```python
from build123d import *

# Parameters (mm, degrees)
BOSS_EXTRUDE1_DEPTH         = 119.0625
F_1_4_20_TAPPED_HOLE2_D     = 5.1054
F_1_4_20_TAPPED_HOLE2_DEPTH = 16.51
F_1_4_20_TAPPED_HOLE2_TIP   = 1.533816902
F_10_32_TAPPED_HOLE1_D      = 4.0386
F_10_32_TAPPED_HOLE1_DEPTH  = 13.6144
F_10_32_TAPPED_HOLE1_TIP    = 1.213317848


with BuildPart() as part:
    # Sketch1 → Boss-Extrude1 (new body)
    with BuildSketch(Plane.XY):
        Polygon((0, 7.332348419), (-6.35, 3.666174209), (-6.35, -3.666174209), (0, -7.332348419), (6.35, -3.666174209), (6.35, 3.666174209), align=None)
    extrude(amount=BOSS_EXTRUDE1_DEPTH)

    # 1/4-20 Tapped Hole2
    with Locations(Plane(origin=(0, 0, 0), x_dir=(-1, 0, 0), z_dir=(0, 0, -1))):
        with Locations((0, 0)):
            Hole(F_1_4_20_TAPPED_HOLE2_D / 2, depth=F_1_4_20_TAPPED_HOLE2_DEPTH)
            with Locations((0, 0, -(F_1_4_20_TAPPED_HOLE2_DEPTH + F_1_4_20_TAPPED_HOLE2_TIP / 2))):  # 118° drill point
                Cone(0, F_1_4_20_TAPPED_HOLE2_D / 2, F_1_4_20_TAPPED_HOLE2_TIP, mode=Mode.SUBTRACT)

    # #10-32 Tapped Hole1
    with Locations(Plane.XY.offset(119.0625)):
        with Locations((0, 0)):
            Hole(F_10_32_TAPPED_HOLE1_D / 2, depth=F_10_32_TAPPED_HOLE1_DEPTH)
            with Locations((0, 0, -(F_10_32_TAPPED_HOLE1_DEPTH + F_10_32_TAPPED_HOLE1_TIP / 2))):  # 118° drill point
                Cone(0, F_10_32_TAPPED_HOLE1_D / 2, F_10_32_TAPPED_HOLE1_TIP, mode=Mode.SUBTRACT)


solid = part.part
```
Geometry check sheet. Reference: the model listing, model coordinates, mm. A direction names the side the tool comes from. Coordinates: 2 decimals unless noted, no trailing zeros. Order: outer loops, then holes, each group sorted by start corner. A loop starts at its lowest first (then second) coordinate and runs counter-clockwise, first axis right, second up.
Item 1: Scan lines: line 1 along X through (y, z) = (0, 116); line 2 along Y through (x, z) = (0, 115); line 3 along X through (y, z) = (0, 11). Record each from-to range of solid material in increasing order.
Item 2: Section check A-A (z = 92.5). Enter the section's corners in (x, y), plus the area to 3 significant figures.
Item 3: Mould release check, pull along X, two halves, no side actions. Record for faces 4 (the conical face through (-0.42, 0.13, 17.78)), 5 (the flat face through (-3.131, 5.525, 58.698)), 6 (the flat face through (3.219, 5.474, 58.698)): released by +X, released by -X, zero draft, split by the parting line, or undercut.
Item 4: Tool access check on faces 1 (the flat face through (1, -2, 119.062)), 2 (the cylindrical face through (2.435, 0.767, 8.371)), 3 (the cylindrical face through (-1.926, 0.607, 112.16)). Record the directions out of +Z, -Z, +X, -X, +Y, -Y that give a thin tool (end or side, any length) a straight path to the whole face; none if there is none.
Item 5: Depth check by flat-ended pin: pin 1 (3 mm diameter, centred on y = 5.5, z = 65, fed in from -X); pin 2 (2 mm diameter, centred on x = -4.5, z = 23.5, fed in from -Y); pin 3 (3 mm diameter, centred on x = 1, z = 32.5, fed in from +Y). Enter the tip coordinate at first touch or a pass-through.
Check sheet entries:
1. line 1: x = -6.35 to -2.02, 2.02 to 6.35
1. line 2: y = -7.33 to -2.02, 2.02 to 7.33
1. line 3: x = -6.35 to -2.55, 2.55 to 6.35
2. outline: (-6.35, -3.67) - (0, -7.33) - (6.35, -3.67) - (6.35, 3.67) - (0, 7.33) - (-6.35, 3.67) - close
2. area: 140 mm2
3. face 4: undercut
3. face 5: released by -X
3. face 6: released by +X
4. face 1: +Z, +X, -X, +Y, -Y
4. face 2: -Z
4. face 3: +Z
5. pin 1: stops at x = -5.77
5. pin 2: stops at y = -5.31
5. pin 3: stops at y = 7.33
